Model file for the job. Use its own axes, mm. Face numbers are marked on the shaded views. A direction names the side the tool comes from. Round coordinates to 2 decimals unless told otherwise and drop trailing zeros. Order: outer loops, then holes, each group sorted by start corner. A loop starts at its lowest first (then second) coordinate and runs counter-clockwise, first axis right, second up. Notation, with made-up numbers: M 38.25,70 L 52.25,70 A17 cw 52.25,79 Z; hole C 75,13.25 d4. An arc over 180 degrees is marked long. Return JSON: item names as keys, results as strings. Group by question number.
Item 1: Slice it at C-C on y = -2. Write the cut outline in (x, z).
Item 2: Probe line 1 along X through (y, z) = (-5.5, 32.5); line 2 along Z through (x, y) = (-9, -28.5); line 3 along Z through (x, y) = (-23.5, -12.5). List the from-to ranges inside material, lowest first.
Item 3: Slice it at B-B on x = -43.5. Write the cut outline in (y, z).
Item 4: Pull direction X, two halves, no side cores. Call the marked faces 3, 4, 5 and 6: pulls with the +X half, pulls with the -X half, needs draft (parallel to the pull), parting line crosses it, or undercut.
Item 5: Pin check, flat tips, straight feed: pin 1 Ø8 at (x, z) = (-7.5, 19) entering from -Y; pin 2 Ø12 at (x, z) = (-26.5, 13.5) entering from -Y; pin 3 Ø8 at (x, y) = (-32.5, -22) entering from +Z; pin 4 Ø4 at (x, y) = (-30, -10) entering from +Z. Stop position of each tip, or through.
Item 6: Which spindle directions (+Z, -Z, +X, -X, +Y, -Y) get a long thin tool onto all of the face, cutting with end or side? Do the marked faces 1 and 2. Say none if no direction does.
Item 7: Slice it at D-D on z = 30.5. Write the cut outline in (x, y).
Item 8: Slice it at A-A on z = 23. Write the cut outline in (x, y).
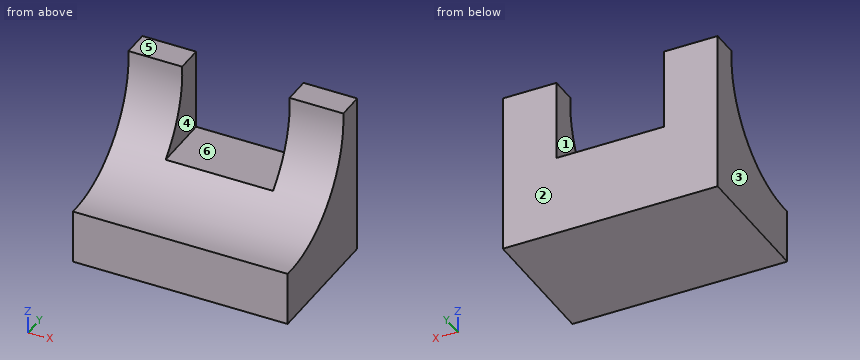
from build123d import *

# Parameters (mm, degrees)
F0_W     = 50.8
F0_H     = 38.1
F1_DEPTH = 31.75
F3_DEPTH = 50.801
F4_W     = 25.4
F4_H     = 19.05
F5_DEPTH = 31.751


with BuildPart() as f1:
    # F0 (on Front) → F1 (new body)
    with BuildSketch(Plane.XZ):
        with Locations((-25.4, 19.05)):
            Rectangle(F0_W, F0_H)
    extrude(amount=F1_DEPTH)

    # F2 (on face) → F3 (cut, through all)
    with BuildSketch(Plane.YZ):
        with BuildLine():
            Line((-31.75, 38.1), (-31.75, 12.7))
            ThreePointArc((-31.75, 12.7), (-13.287516, 19.637516), (-6.35, 38.1))
            Line((-6.35, 38.1), (-31.75, 38.1))
        make_face()
    extrude(amount=-F3_DEPTH, mode=Mode.SUBTRACT)

    # F4 (on face) → F5 (cut, through all)
    with BuildSketch(Plane(origin=(0, 0, 0), x_dir=(-1, 0, 0), z_dir=(0, 1, 0))):
        with Locations((25.4, 28.575)):
            Rectangle(F4_W, F4_H)
    extrude(amount=-F5_DEPTH, mode=Mode.SUBTRACT)


solid = f1.part
Output values:
{
 "1": {"outline": "M -50.8,0 L 0,0 L 0,38.1 L -12.7,38.1 L -12.7,19.05 L -38.1,19.05 L -38.1,38.1 L -50.8,38.1 Z"},
 "2": {"line 1": "-50.8 to -38.1, -12.7 to 0", "line 2": "0 to 12.71", "line 3": "0 to 19.05"},
 "3": {"outline": "M -31.75,0 L 0,0 L 0,38.1 L -6.35,38.1 A23.87 cw -31.75,12.7 Z"},
 "4": {"face 3": "pulls with the -X half", "face 4": "undercut", "face 5": "needs draft", "face 6": "undercut"},
 "5": {"pin 1": "y = -19.83", "pin 2": "y = -31.75", "pin 3": "z = 15.98", "pin 4": "z = 19.05"},
 "6": {"face 1": "+Z, +Y, -Y", "face 2": "+Z, -Z, +X, -X, +Y"},
 "7": {"outline": "M -50.8,-7.07 L -38.1,-7.07 L -38.1,0 L -50.8,0 Z; M -12.7,-7.07 L 0,-7.07 L 0,0 L -12.7,0 Z"},
 "8": {"outline": "M -50.8,-10.49 L -38.1,-10.49 L -38.1,0 L -50.8,0 Z; M -12.7,-10.49 L 0,-10.49 L 0,0 L -12.7,0 Z"}
}
